Could you check a few things on this model? Use its own coordinates, in mm. A direction names the side the tool comes from. Round coordinates to 2 decimals unless told otherwise and drop trailing zeros. Write each loop counter-clockwise with the first axis right and the second up, starting at its lowest first coordinate (ties: lowest second). Pieces come first, ordered by that corner, then holes. Notation, with made-up numbers: (40.25, 56) - (46.25, 56) arc R32 ccw to (46.25, 89) - close; hole circle Ø6 at (-24, 49.25). An arc over 180 degrees is marked (long way). Write each question's results on one line, items separated by ' | '. Start each with the question number.
(1) Thinking about a two-plate mould opening in Y: for faces 4 (the cylindrical face through (55, 0, 2)), 5 (the cylindrical face through (-0.035, 12.669, -0.526)), 6 (the cylindrical face through (-45.042, -1.247, 2.465)), 7 (the flat face through (12, 0, 0)), which applies, +Y half, -Y half, draft (parallel to the pull), parting line (faces both ways), or undercut?
(2) Imagine slicing it at B-B on y = 0. Write out the boundary of the cut face in (x, z), then the cut area to 3 significant figures.
(3) Imagine slicing it at A-A on x = 48. Write out the boundary of the cut face in (y, z).
(4) On a 3-axis mill with a long thin cutter (end or side, diameter ignored), from which of +Z, -Z, +X, -X, +Y, -Y can I reach the whole of each face in a straight line? I mean faces 1 (the flat face through (2.5, 7, 0)), 2 (the cylindrical face through (-21.506, -0.264, -19.72)), 3 (the flat face through (-0.04, 1.87, -2.42)). Say none if no direction works.
(5) Imagine slicing it at D-D on x = 5.5. Write out the boundary of the cut face in (y, z), then the cut area to 3 significant figures.
(6) Please list where these lines run through material, in increasing order: line 1 (Z direction, x = 0.6, y = 11); line 2 (X direction, y = 0, z = -4.5); line 3 (Y direction, x = -49, z = 1.4). Write a range as [from, to].
(7) Imagine slicing it at C-C on z = -11.5. Write out the boundary of the cut face in (x, y).
(8) For P1, Ø6, axis at x = -45.5, y = 2, coming from the -Z side; P2, Ø5, axis at y = -0.5, z = -21.5, coming from the -X side; P3, Ø3, axis at y = 9.5, z = -8, coming from the +X side; P4, Ø1, axis at y = 1.5, z = -3.5, coming from the -X side, each with a flat end and sliding along its axis, tell me the tip position at first contact or that it passes through.
Autodesk Inventor part; units mm, degrees
ref_plane "YZ Plane" through (0, 0, 0) normal (1, 0, 0) x (0, 1, 0)
ref_plane "XZ Plane" through (0, 0, 0) normal (0, 1, 0) x (-1, 0, 0)
ref_plane "XY Plane" through (0, 0, 0) normal (0, 0, 1) x (1, 0, 0)
sketch "Sketch1" plane through (0, 0, 0) normal (0, 0, 1) x (1, 0, 0)
  line L0 (-49, 0) -> (49, 0) construction
  line L1 (-49, -6) -> (49, -6)
  line L2 (49, 6) -> (-49, 6)
  arc A0 (-49, 6) -> (-49, -6) centre (-49, 0) ccw
  arc A1 (49, -6) -> (49, 6) centre (49, 0) ccw
  circle A2 centre (49, 0) radius 4.15
  circle A3 centre (-49, 0) radius 4.15
  point P0 (0, 0)
  dimension "d0" = 49
  dimension "d1" = 12
  dimension "d2" = 8.3
  dimension "d3" = 8.3
extrude "Extrusion1" add sketch "Sketch1" along normal blind 5
sketch "Sketch2" plane through (0, 0, 0) normal (1, 0, 0) x (0, 1, 0)
  circle A0 centre (11, 0) radius 1.75
  circle A1 centre (11, 0) radius 5
  line L0 (6, 5) -> (-6, 5)
  line L1 (6, 5) -> (11, 5)
  line L2 (9.5294, -4.7788) -> (-6, 0)
  line L3 (-6, 0) -> (6, 0)
  line L4 (6, 0) -> (6, 5)
  line L5 (-6, 5) -> (6, 5)
  line L6 (-6, 0) -> (-6, 5)
  line L7 (6, 0) -> (6, 5)
  point P0 (0, 0)
  point P1 (-6, 0)
  dimension "d6" = 3.5
  dimension "d7" = 10
extrude "Extrusion2" add sketch "Sketch2" along normal mid plane 5 contours A1 | A1 L4 L1 | L2 L3 A1
sketch "Sketch3" plane through (0, 0, 0) normal (0, 0, -1) x (-1, 0, 0)
  circle A0 centre (-27.5, 0) radius 6
  line L0 (-49, 6) -> (-2.5, 6)
  line L1 (2.5, -6) -> (-2.5, -6)
  line L2 (0, -6) -> (0, -9.8516)
  line L3 (-2.5, -6) -> (-49, -6)
  line L4 (-2.5, -6) -> (-2.5, 9.5294)
  circle A1 centre (27.5, 0) radius 6
  point P0 (0, 0)
  dimension "d10" = 25
extrude "Extrusion3" add sketch "Sketch3" along normal blind 40 contours A0 | A1
properties part number "Support slider_3DPrint"
Response:
1) face 4: parting line | face 5: undercut | face 6: undercut | face 7: draft
2) outline: (-55, 0) - (-53.15, 0) - (-53.15, 5) - (-55, 5) - close; (-44.85, 0) - (-33.5, 0) - (-33.5, -40) - (-21.5, -40) - (-21.5, 0) - (-2.5, 0) - (-2.5, -1.85) - (2.5, -1.85) - (2.5, 0) - (21.5, 0) - (21.5, -40) - (33.5, -40) - (33.5, 0) - (44.85, 0) - (44.85, 5) - (-44.85, 5) - close; (53.15, 0) - (55, 0) - (55, 5) - (53.15, 5) - close | area: 1,440 mm²
3) outline: (-6, 0) - (-4.03, 0) - (-4.03, 5) - (-6, 5) - close; (4.03, 0) - (6, 0) - (6, 5) - (4.03, 5) - close
4) face 1: -Z, +Y | face 2: -Z | face 3: -Z, -Y
5) outline: (-6, 0) - (6, 0) - (6, 5) - (-6, 5) - close | area: 60.0 mm²
6) line 1: [-5, -1.75], [1.75, 5] | line 2: [-33.5, -21.5], [21.5, 33.5] | line 3: [-6, -4.15], [4.15, 6]
7) outline: circle Ø12 at (-27.5, 0); circle Ø12 at (27.5, 0)
8) P1: z = 0 | P2: x = -33.5 | P3: through | P4: x = -33.42
